Geometry: final body of the model. Coordinates: model frame, mm. Face numbers are marked on the shaded views. A direction names the side the tool comes from. Coordinates: 2 decimals unless noted, no trailing zeros. Loops run counter-clockwise (first coordinate to the right, second up) from the corner with the lowest first, then second, coordinate; pieces in that order, holes last. Notation, with made-up numbers: M -11,17.25 L -4,17.25 A36 ccw -4,54.25 Z; hole C 25.25,-10.75 d6. An arc over 180 degrees is marked long. Write item = value, one per line. Start each with the question number.
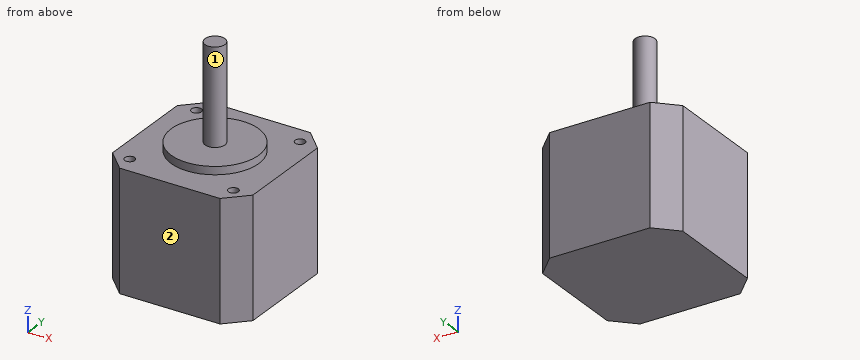
```python
from build123d import *

# Parameters (mm, degrees)
F0_W     = 35.2
F0_H     = 35.2
F1_DEPTH = 30
F2_SIZE  = 5
F5_R     = 1.25
F6_DEPTH = 5


with BuildPart() as f1:
    # F0 (on Top) → F1 (new body)
    with BuildSketch(Plane.XY):
        Rectangle(F0_W, F0_H)
    extrude(amount=F1_DEPTH)

    # F2
    f2_edges = [f1.edges().sort_by_distance(p)[0] for p in [
        (17.6, -17.6, 15),
        (-17.6, -17.6, 15),
        (-17.6, 17.6, 15),
        (17.6, 17.6, 15),
    ]]
    chamfer(f2_edges, length=F2_SIZE)

    # F3 (on Right) → F4 (revolve)
    with BuildSketch(Plane.YZ):
        Polygon((-11, 30), (0, 30), (0, 56), (-2.5, 56), (-2.5, 32), (-11, 32), align=None)
    revolve(axis=Axis((0, 0, 43), (0, 0, 1)))

    # F5 (on face) → F6 (cut)
    with BuildSketch(Plane.XY.offset(30)):
        with Locations((-13, 13)):
            Circle(F5_R)
        with Locations((13, 13)):
            Circle(F5_R)
        with Locations((13, -13)):
            Circle(F5_R)
        with Locations((-13, -13)):
            Circle(F5_R)
    extrude(amount=-F6_DEPTH, mode=Mode.SUBTRACT)


solid = f1.part
```
Item 1: Section query B-B (y = 0). Return the cut outline in (x, z).
Item 2: Section query A-A (z = 27). Return the cut outline in (x, y).
Item 3: Section query C-C (z = 8). Return the cut outline in (x, y), plus the area to 3 significant figures.
Item 4: First-contact query: pin 1 (2 mm diameter, centred on x = 13.5, y = 13.5, fed in from +Z); pin 2 (2 mm diameter, centred on x = -13, y = -13, fed in from +Z); pin 3 (12 mm diameter, centred on x = 6.5, y = -11.5, fed in from +Z); pin 4 (3 mm diameter, centred on y = 5.5, z = 41, fed in from +X) (3 decimals). Flat tips, straight axial feed; report the tip coordinate or a pass-through.
Item 5: Line query: line 1 (Y direction, x = -13, z = 27.6); line 2 (Z direction, x = 4, y = 11); line 3 (Z direction, x = -5.5, y = 6). Output: solid intervals per line, ascending. Write a range as from..to.
Item 6: Reachability of the marked faces 1 and 2 from +Z, -Z, +X, -X, +Y, -Y: full face, straight path, thin tool, end or side. Return the list, or none.
Verdict:
q1.outline = M -17.6,0 L 17.6,0 L 17.6,30 L 11,30 L 11,32 L 2.5,32 L 2.5,56 L -2.5,56 L -2.5,32 L -11,32 L -11,30 L -17.6,30 Z
q2.outline = M -17.6,-12.6 L -12.6,-17.6 L 12.6,-17.6 L 17.6,-12.6 L 17.6,12.6 L 12.6,17.6 L -12.6,17.6 L -17.6,12.6 Z; hole C -13,-13 d2.5; hole C -13,13 d2.5; hole C 13,-13 d2.5; hole C 13,13 d2.5
q3.outline = M -17.6,-12.6 L -12.6,-17.6 L 12.6,-17.6 L 17.6,-12.6 L 17.6,12.6 L 12.6,17.6 L -12.6,17.6 L -17.6,12.6 Z
q3.area = 1,190 mm2
q4.pin_1 = 30
q4.pin_2 = 25
q4.pin_3 = 32
q4.pin_4 = through
q5.line_1 = -17.2..-14.25, -11.75..11.75, 14.25..17.2
q5.line_2 = 0..30
q5.line_3 = 0..32
q6.face_1 = +Z
q6.face_2 = +Z, -Z, +X, -X, -Y
